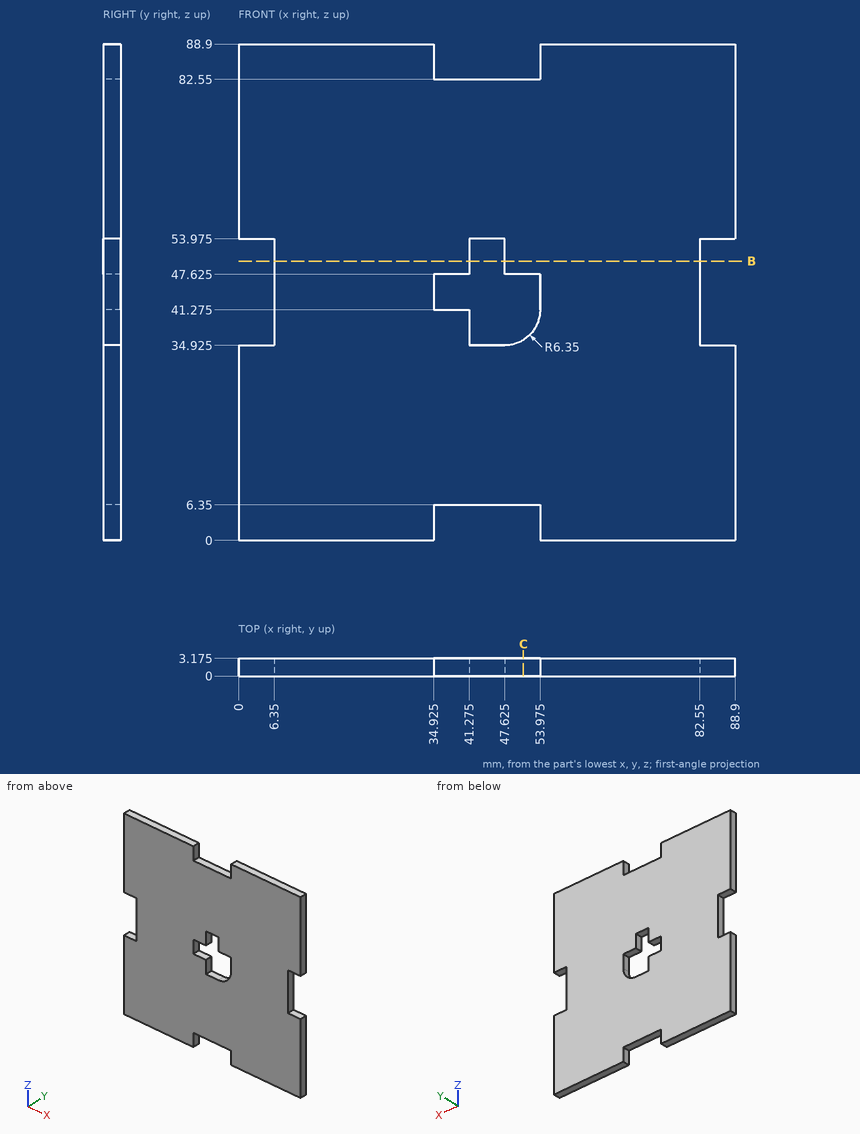
Check sheet for the drawn part. Datum: minimum x, y, z corner. Units: mm. Round coordinates to 2 decimals unless told otherwise and drop trailing zeros. Write each loop counter-clockwise with the first axis right and the second up, starting at its lowest first coordinate (ties: lowest second). Pieces come first, ordered by that corner, then holes. Notation, with made-up numbers: (41, 63.25) - (71, 63.25) arc R9 ccw to (71, 70.25) - close; hole circle Ø3 at (-31, 88). An arc over 180 degrees is marked (long way). Return JSON: item names as keys, results as strings.
Q1. Cross-section at B-B (z = 50). Record the boundary of the cut face in (x, y) (3 decimals), then the cut area to 3 significant figures.
Returned:
{"outline": "(6.35, 0) - (41.275, 0) - (41.275, 3.175) - (6.35, 3.175) - close; (47.625, 0) - (82.55, 0) - (82.55, 3.175) - (47.625, 3.175) - close", "area": "222 mm²"}
Q2. Depth check by flat-ended pin: P1, Ø1, axis at y = 2.5, z = 45, coming from the -X side; P2, Ø1, axis at y = 1.5, z = 37.5, coming from the +X side. Enter the tip coordinate at first touch or a pass-through.
Returned:
{"P1": "stops at x = 6.35", "P2": "stops at x = 82.55"}
Q3. Cross-section at C-C (x = 51). Record the boundary of the cut face in (y, z) (3 decimals), then the cut area to 3 significant figures.
Returned:
{"outline": "(0, 6.35) - (3.175, 6.35) - (3.175, 35.896) - (0, 35.896) - close; (0, 47.625) - (3.175, 47.625) - (3.175, 82.55) - (0, 82.55) - close", "area": "205 mm²"}
Q4. Scan lines: L1, parallel to X at y = 1.4, z = 83 (3 decimals); L2, parallel to Z at x = 39, y = 1.4 (3 decimals). Record each from-to range of solid material in increasing order. Write a range as from..to.
Returned:
{"L1": "x = 0..34.925, 53.975..88.9", "L2": "z = 6.35..41.275, 47.625..82.55"}
